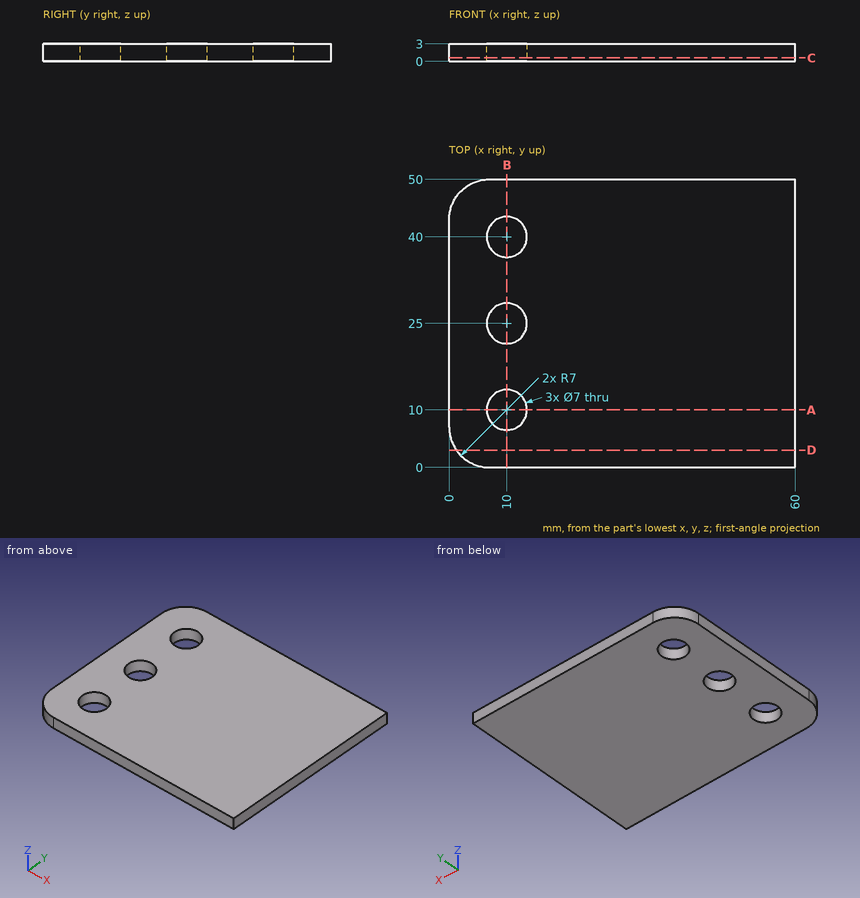
For this review, use the dimensioned drawing (mm, ordinates from the lowest corner) and the shaded views. Round coordinates to 2 decimals unless told otherwise and drop trailing zeros. Order: outer loops, then holes, each group sorted by start corner. A loop starts at its lowest first (then second) coordinate and runs counter-clockwise, first axis right, second up.
1) Consider section D-D (y = 3). State the section outline as (x, z) points.
The answers:
outline: (1.26, 0) - (60, 0) - (60, 3) - (1.26, 3) - close
2) Consider section A-A (y = 10). State the section outline as (x, z) points, plus the area to 3 significant figures.
The answers:
outline: (0, 0) - (6.5, 0) - (6.5, 3) - (0, 3) - close; (13.5, 0) - (60, 0) - (60, 3) - (13.5, 3) - close
area: 159 mm2
3) Consider section C-C (z = 0.6). State the section outline as (x, y) points, plus the area to 3 significant figures.
The answers:
outline: (0, 7) arc R7 ccw to (7, 0) - (60, 0) - (60, 50) - (7, 50) arc R7 ccw to (0, 43) - close; hole circle Ø7 at (10, 10); hole circle Ø7 at (10, 25); hole circle Ø7 at (10, 40)
area: 2,860 mm2
4) For L1, parallel to Y at x = 10, z = 1.7; L2, parallel to Y at x = 11.5, z = 1.5; L3, parallel to X at y = 39, z = 0.7, list the stretches that pass through material, from the lowest coordinate up.
The answers:
L1: y = 0 to 6.5, 13.5 to 21.5, 28.5 to 36.5, 43.5 to 50
L2: y = 0 to 6.84, 13.16 to 21.84, 28.16 to 36.84, 43.16 to 50
L3: x = 0 to 6.65, 13.35 to 60
5) Consider section B-B (x = 10). State the section outline as (y, z) points, plus the area to 3 significant figures.
The answers:
outline: (0, 0) - (6.5, 0) - (6.5, 3) - (0, 3) - close; (13.5, 0) - (21.5, 0) - (21.5, 3) - (13.5, 3) - close; (28.5, 0) - (36.5, 0) - (36.5, 3) - (28.5, 3) - close; (43.5, 0) - (50, 0) - (50, 3) - (43.5, 3) - close
area: 87.0 mm2
